The listing builds one solid part. Answer for the finished solid, in the listing's coordinates (mm). Face numbers are marked on the shaded views. A direction names the side the tool comes from. Coordinates: 2 decimals unless noted, no trailing zeros. Loops run counter-clockwise (first coordinate to the right, second up) from the corner with the lowest first, then second, coordinate; pieces in that order, holes last. Notation, with made-up numbers: (19, 86) - (76, 86) arc R18 ccw to (76, 101) - close; hole circle Ø8 at (-10.75, 33). An arc over 180 degrees is marked (long way). Put each result on its own line as item: value.
```python
from build123d import *

# Parameters (mm, degrees)
L_BASE_DEPTH                                = 12.7
SKETCH3_W                                   = 44.45
SKETCH3_H                                   = 25.4
RECTANGULAR_EXTRUDE_DEPTH                   = 10.5664
SKETCH4_W                                   = 11.1125
SKETCH4_H                                   = 25.4
FORK_EXTRUDE_DEPTH                          = 29.3624
SKETCH6_W                                   = 38.354
SKETCH6_H                                   = 3.302
F_4_EXPANSION_INSERT_RECESSES_1_D           = 3.2639
F_4_EXPANSION_INSERT_RECESSES_1_DEPTH       = 12.7
F_4_EXPANSION_INSERT_RECESSES_1_CBORE_D     = 3.96875
F_4_EXPANSION_INSERT_RECESSES_1_CBORE_DEPTH = 4.7625
F_4_EXPANSION_INSERT_RECESSES_1_TIP         = 0.980574487
F_4_EXPANSION_INSERT_RECESSES_2_D           = 3.2639
F_4_EXPANSION_INSERT_RECESSES_2_DEPTH       = 9.525
F_4_EXPANSION_INSERT_RECESSES_2_CBORE_D     = 3.96875
F_4_EXPANSION_INSERT_RECESSES_2_CBORE_DEPTH = 4.7625
F_4_EXPANSION_INSERT_RECESSES_2_TIP         = 0.980574487
L_BASE_FILLET_R                             = 6.35
FORK_FILLET_R                               = 3.175
INSTALLATION_CHAMFERS_1_SIZE                = 0.508
INSTALLATION_CHAMFERS_2_SIZE                = 0.508
PRINT_BED_CHAMFER_SIZE                      = 0.508


with BuildPart() as part:
    # Sketch1 → L-Base (new body)
    with BuildSketch(Plane(origin=(0, 0, 0), x_dir=(1, 0, 0), z_dir=(0, 1, 0))):
        Polygon((0, 0), (44.45, 0), (44.45, 25.4), (20.066, 25.4), (20.066, 39.116), (0, 39.116), align=None)
    extrude(amount=L_BASE_DEPTH)

    # Sketch3 → Rectangular Extrude (add)
    with BuildSketch(Plane(origin=(0, 12.7, 0), x_dir=(1, 0, 0), z_dir=(0, 1, 0))):
        with Locations((22.225, 12.7)):
            Rectangle(SKETCH3_W, SKETCH3_H)
    extrude(amount=RECTANGULAR_EXTRUDE_DEPTH)

    # Sketch4 → Fork Extrude (add)
    with BuildSketch(Plane(origin=(0, 23.2664, 0), x_dir=(1, 0, 0), z_dir=(0, 1, 0))):
        with Locations((5.55625, 12.7)):
            Rectangle(SKETCH4_W, SKETCH4_H)
        with Locations((38.89375, 12.7)):
            Rectangle(SKETCH4_W, SKETCH4_H)
    extrude(amount=FORK_EXTRUDE_DEPTH)

    # Sketch6 → Shaft Recess (revolve, cut)
    with BuildSketch(Plane(origin=(0, 52.6288, 0), x_dir=(1, 0, 0), z_dir=(0, 1, 0))):
        with Locations((22.225, 11.049)):
            Rectangle(SKETCH6_W, SKETCH6_H)
    revolve(axis=Axis((0, 52.6288, -12.7), (1, 0, 0)), mode=Mode.SUBTRACT)

    # #4 Expansion Insert Recesses #1
    with Locations(Plane(origin=(0, 52.6288, 0), x_dir=(1, 0, 0), z_dir=(0, 1, 0))):
        with Locations((5.55625, 20.701), (5.55625, 4.699), (38.89375, 20.701), (38.89375, 4.699)):
            CounterBoreHole(F_4_EXPANSION_INSERT_RECESSES_1_D / 2, F_4_EXPANSION_INSERT_RECESSES_1_CBORE_D / 2, F_4_EXPANSION_INSERT_RECESSES_1_CBORE_DEPTH, depth=F_4_EXPANSION_INSERT_RECESSES_1_DEPTH)
            with Locations((0, 0, -(F_4_EXPANSION_INSERT_RECESSES_1_DEPTH + F_4_EXPANSION_INSERT_RECESSES_1_TIP / 2))):  # 118° drill point
                Cone(0, F_4_EXPANSION_INSERT_RECESSES_1_D / 2, F_4_EXPANSION_INSERT_RECESSES_1_TIP, mode=Mode.SUBTRACT)

    # #4 Expansion Insert Recesses #2
    with Locations(Plane(origin=(0, 0, 0), x_dir=(-1, 0, 0), z_dir=(0, -1, 0))):
        with Locations((-10.033, 10.033), (-28.956, 10.033), (-10.033, 28.956)):
            CounterBoreHole(F_4_EXPANSION_INSERT_RECESSES_2_D / 2, F_4_EXPANSION_INSERT_RECESSES_2_CBORE_D / 2, F_4_EXPANSION_INSERT_RECESSES_2_CBORE_DEPTH, depth=F_4_EXPANSION_INSERT_RECESSES_2_DEPTH)
            with Locations((0, 0, -(F_4_EXPANSION_INSERT_RECESSES_2_DEPTH + F_4_EXPANSION_INSERT_RECESSES_2_TIP / 2))):  # 118° drill point
                Cone(0, F_4_EXPANSION_INSERT_RECESSES_2_D / 2, F_4_EXPANSION_INSERT_RECESSES_2_TIP, mode=Mode.SUBTRACT)

    # L-Base Fillet
    l_base_fillet_edges = [part.edges().sort_by_distance(p)[0] for p in [
        (10.033, 12.7, -39.116),
        (10.033, 12.7, -25.4),
        (20.066, 6.35, -25.4),
    ]]
    fillet(l_base_fillet_edges, radius=L_BASE_FILLET_R)

    # Fork Fillet
    fork_fillet_edges = [part.edges().sort_by_distance(p)[0] for p in [
        (33.3375, 23.2664, -12.7),
        (11.1125, 23.2664, -12.7),
    ]]
    fillet(fork_fillet_edges, radius=FORK_FILLET_R)

    # Installation Chamfers #1
    installation_chamfers_1_edges = [part.edges().sort_by_distance(p)[0] for p in [
        (36.909375, 52.6288, -4.699),
        (36.909375, 52.6288, -20.701),
        (3.571875, 52.6288, -4.699),
        (3.571875, 52.6288, -20.701),
    ]]
    chamfer(installation_chamfers_1_edges, length=INSTALLATION_CHAMFERS_1_SIZE)

    # Installation Chamfers #2
    installation_chamfers_2_edges = [part.edges().sort_by_distance(p)[0] for p in [
        (30.940375, 0, -10.033),
        (12.017375, 0, -10.033),
        (12.017375, 0, -28.956),
    ]]
    chamfer(installation_chamfers_2_edges, length=INSTALLATION_CHAMFERS_2_SIZE)

    # Print Bed Chamfer
    print_bed_chamfer_edges = [part.edges().sort_by_distance(p)[0] for p in [
        (20.066, 0, -35.433),
        (21.925871939, 0, -27.259871939),
        (10.033, 0, -39.116),
        (35.433, 0, -25.4),
        (44.45, 0, -12.7),
        (22.225, 0, 0),
        (0, 0, -19.558),
    ]]
    chamfer(print_bed_chamfer_edges, length=PRINT_BED_CHAMFER_SIZE)


solid = part.part
```
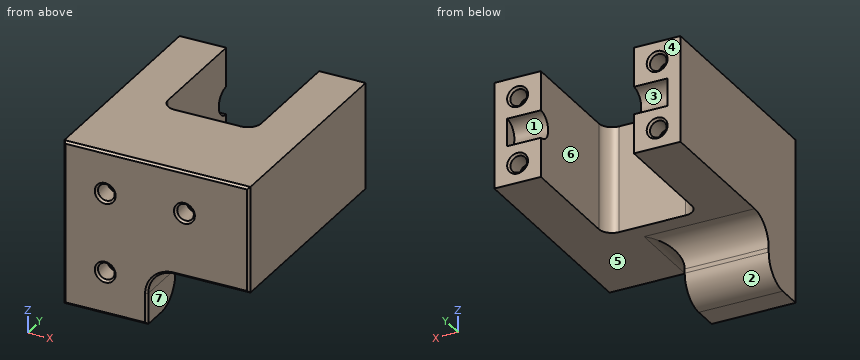
1) The part is cut by section A-A (y = 34). Give the vertices of the cut face in (x, z), and give its area (3 significant figures).
Found:
outline: (0, -25.4) - (11.11, -25.4) - (11.11, 0) - (0, 0) - close; (33.34, -25.4) - (44.45, -25.4) - (44.45, 0) - (33.34, 0) - close
area: 565 mm^2
2) Each of these flat-tipped pins is pushed along its axis until it touches: pin 1 (5 mm diameter, centred on x = 28.956, z = -10.033, fed in from +Y); pin 2 (2.5 mm diameter, centred on x = 38.89, z = -20.7, fed in from +Y); pin 3 (3.5 mm diameter, centred on y = 7.5, z = -36.5, fed in from +X). Where does it stop, or does it pass through?
Found:
pin 1: stops at y = 23.54
pin 2: stops at y = 39.7
pin 3: stops at x = 20.07
3) For the marked faces 5, 6 and 7, determine the directions among +Z, -Z, +X, -X, +Y, -Y from which every point of the face is accessible in a straight line to the end or side of a thin tool.
Found:
face 5: -Z, +X, +Y
face 6: +Z, -Z, +Y
face 7: -Z, +X, +Y, -Y
4) For a pull along Z with two mould halves and no side action, classify the marked faces 1, 2, 3 and 4 as pulls with the +Z half, pulls with the -Z half, needs draft (parallel to the pull), parting line crosses it, or undercut.
Found:
face 1: undercut
face 2: pulls with the -Z half
face 3: undercut
face 4: needs draft
5) Straight lines are drawn through the part: L1, parallel to X at y = 47, z = -11; L2, parallel to Z at x = 40, y = 48; L3, parallel to Z at x = 2, y = 29. For each, find the intervals that lie inside material, in ascending order. Write a range as [from, to].
Found:
L1: x = [0, 11.11], [33.34, 44.45]
L2: z = [-25.4, -22.35], [-19.05, -6.35], [-3.05, 0]
L3: z = [-25.4, 0]
